Model file for the job. Use its own axes, mm. Face numbers are marked on the shaded views. A direction names the side the tool comes from. Give positions to 0.01 mm unless a question says otherwise; leave off trailing zeros. Write each loop counter-clockwise with the first axis right and the second up, starting at its lowest first coordinate (ties: lowest second). Pieces come first, ordered by that corner, then holes.
```python
from build123d import *

# Parameters (mm, degrees)
F0_W          = 65
F0_H          = 12.5
F0_R          = 1.5
F1_DEPTH      = 2.5
F2_W          = 65
F2_H          = 2.5
F3_DEPTH      = 10
F4_R          = 2
F5_DEPTH      = 3
F5_DEPTH_BACK = 3


with BuildPart() as f1:
    # F0 (on Top) → F1 (new body)
    with BuildSketch(Plane.XY):
        Rectangle(F0_W, F0_H)
        with Locations((-17.5, -1.25)):
            Circle(F0_R, mode=Mode.SUBTRACT)
        with Locations((17.5, -1.25)):
            Circle(F0_R, mode=Mode.SUBTRACT)
    extrude(amount=F1_DEPTH)

    # F2 (on face) → F3 (join)
    with BuildSketch(Plane.XY.offset(2.5)):
        with Locations((0, 5)):
            Rectangle(F2_W, F2_H)
    extrude(amount=F3_DEPTH)

    # F4 (on Right) → F5 (join, two sides)
    with BuildSketch(Plane.YZ) as f5_sk:
        with BuildLine():
            Line((6.25, 12.5), (6.25, 0))
            Line((6.25, 0), (31.25, 0))
            ThreePointArc((31.25, 0), (37.5, 6.25), (31.25, 12.5))
            Line((31.25, 12.5), (6.25, 12.5))
        make_face()
        with Locations((31.25, 6.25)):
            Circle(F4_R, mode=Mode.SUBTRACT)
    extrude(amount=F5_DEPTH)
    extrude(f5_sk.sketch, amount=-F5_DEPTH_BACK)


solid = f1.part
```
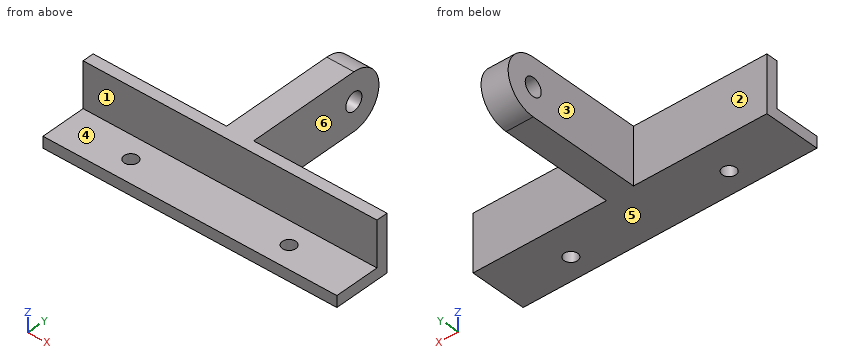
1. Slice it at C-C, the plane z = 6.25. Write the cut outline in (x, y), and give its area (3 significant figures).
Calculated:
outline: (-32.5, 3.75) - (32.5, 3.75) - (32.5, 6.25) - (3, 6.25) - (3, 29.25) - (-3, 29.25) - (-3, 6.25) - (-32.5, 6.25) - close; (-3, 33.25) - (3, 33.25) - (3, 37.5) - (-3, 37.5) - close
area: 326 mm2
2. Slice it at A-A, the plane y = -1.25. Write the cut outline in (x, z).
Calculated:
outline: (-32.5, 0) - (-19, 0) - (-19, 2.5) - (-32.5, 2.5) - close; (-16, 0) - (16, 0) - (16, 2.5) - (-16, 2.5) - close; (19, 0) - (32.5, 0) - (32.5, 2.5) - (19, 2.5) - close
3. Probe probe 1 along Y at (x, z) = (17.5, 0.85); probe 2 along Z at (x, y) = (1, 31); probe 3 along Y at (x, z) = (12.5, 5.5). List the from-to ranges inside material, lowest first.
Calculated:
probe 1: y = -6.25 to -2.75, 0.25 to 6.25
probe 2: z = 0 to 4.27, 8.23 to 12.5
probe 3: y = 3.75 to 6.25
4. Slice it at D-D, the plane x = -2. Write the cut outline in (y, z).
Calculated:
outline: (-6.25, 0) - (31.25, 0) arc R6.25 ccw to (31.25, 12.5) - (3.75, 12.5) - (3.75, 2.5) - (-6.25, 2.5) - close; hole circle Ø4 at (31.25, 6.25)
5. Slice it at B-B, the plane x = 17.5. Write the cut outline in (y, z).
Calculated:
outline: (-6.25, 0) - (-2.75, 0) - (-2.75, 2.5) - (-6.25, 2.5) - close; (0.25, 0) - (6.25, 0) - (6.25, 12.5) - (3.75, 12.5) - (3.75, 2.5) - (0.25, 2.5) - close
6. Which spindle directions (+Z, -Z, +X, -X, +Y, -Y) get a long thin tool onto all of the face, cutting with end or side? Do the marked faces 4, 5 and 6. Say none if no direction does.
Calculated:
face 4: +Z, +X, -X, -Y
face 5: -Z, +X, -X, +Y, -Y
face 6: +Z, -Z, +X, +Y
7. Pull direction Y, two halves, no side cores. Call the marked faces 1, 2 and 3: +Y half, -Y half, draft (parallel to the pull), parting line (faces both ways), or undercut.
Calculated:
face 1: -Y half
face 2: +Y half
face 3: draft
8. Pin check, flat tips, straight feed: P1, Ø1.5, axis at y = 19.5, z = 10.5, coming from the +X side; P2, Ø8, axis at x = 4.5, y = -2.5, coming from the +Z side; P3, Ø3, axis at x = 5.5, z = 6, coming from the -Y side. Stop position of each tip, or through.
Calculated:
P1: stops at x = 3
P2: stops at z = 2.5
P3: stops at y = 3.75
